Here's how the part is built. I have some questions about the finished solid (model axes, mm). A direction names the side the tool comes from. Coordinates: 2 decimals unless noted, no trailing zeros. Write each loop counter-clockwise with the first axis right and the second up, starting at its lowest first coordinate (ties: lowest second). Pieces come first, ordered by that corner, then holes.
Item 1: If I drill on line 1 (Y direction, x = -47, z = 120); line 2 (Z direction, x = -17, y = -6); line 3 (X direction, y = 11.5, z = 77.5), over which ranges is the centre line in solid material (lowest first)?
Item 2: I'm going to push flat-ended pins straight in: pin 1 Ø6 at (x, z) = (-8, -34) entering from +Y; pin 2 Ø4.5 at (x, z) = (-44.5, 119.5) entering from -Y; pin 3 Ø4.5 at (y, z) = (-14, -119.5) entering from -X; pin 4 Ø14.5 at (x, y) = (-12.5, -17) entering from -Z. Where does each tip first touch, or does it pass through?
Item 3: If we section it at B-B (x = -36.5): Please give me the cut outline in (y, z).
Item 4: If we section it at D-D (z = 7): Please give me the cut outline in (x, y), then the cut area to 3 significant figures.
Item 5: For faces 5 (the face through (-30, 32, -2)), 6 (the face through (-27, 32, -2)), 7 (the face through (2, -19, 119.25)), which set-ups out of +Z, -Z, +X, -X, +Y, -Y let a thin tool reach every point of the face, with its end or its side?
Item 6: If we section it at A-A (y = 17.5): Please give me the cut outline in (x, z).
Item 7: We'd pull the mould along Y, two halves only. Please class faces 1 (the face through (2, -19, 122.25)), 2 (the face through (14.1, -13.9, 120.8)), 3 (the face through (2, 0, -2)), 4 (the face through (-29, 60, 1)): +Y half, -Y half, draft (parallel to the pull), parting line (faces both ways), or undercut.
Item 8: If we section it at C-C (x = -12.5): Please give me the cut outline in (y, z).
from build123d import *

# Parameters (mm, degrees)
SKETCH1_W                      = 60
SKETCH1_H                      = 244.5
BASE_FLANGE1_DEPTH             = 3
EDGE_FLANGE1_STRIP_W           = 14
EDGE_FLANGE1_STRIP_H           = 3
EDGE_FLANGE1_STRIP_CUT_DEPTH   = 244.5
EDGE_FLANGE1_DEPTH             = 244.5
EDGE_FLANGE2_STRIP_W           = 14
EDGE_FLANGE2_STRIP_H           = 3
EDGE_FLANGE2_STRIP_CUT_DEPTH   = 56
EDGE_FLANGE2_STRIP_2_W         = 14
EDGE_FLANGE2_STRIP_2_H         = 3
EDGE_FLANGE2_STRIP_CUT_2_DEPTH = 56
EDGE_FLANGE2_STRIP_3_W         = 14
EDGE_FLANGE2_STRIP_3_H         = 3
EDGE_FLANGE2_STRIP_CUT_3_DEPTH = 56
EDGE_FLANGE2_STRIP_4_W         = 14
EDGE_FLANGE2_STRIP_4_H         = 3
EDGE_FLANGE2_STRIP_CUT_4_DEPTH = 56
EDGE_FLANGE2_DEPTH             = 56
EDGE_FLANGE2_BEND_DEPTH        = 56
EDGE_FLANGE2_BEND_2_DEPTH      = 56
EDGE_FLANGE2_BEND_3_DEPTH      = 56
SKETCH18_R                     = 4.6
EXTRUDE1_DEPTH                 = 261.517273899


# Sheet-metal steps are written as plain solids
with BuildPart() as part:
    # Sketch1 → Base-Flange1 (new body)
    with BuildSketch(Plane(origin=(0, 0, 0), x_dir=(1, 0, 0), z_dir=(0, 1, 0))):
        Rectangle(SKETCH1_W, SKETCH1_H)
    extrude(amount=BASE_FLANGE1_DEPTH)

    # Edge-Flange1 strip (across the edge) → Edge-Flange1 strip cut (cut)
    with BuildSketch(Plane(origin=(-30, 3, -122.25), x_dir=(1, 0, 0), z_dir=(0, 0, 1))):
        with Locations((-3, -1.5)):
            Rectangle(EDGE_FLANGE1_STRIP_W, EDGE_FLANGE1_STRIP_H)
    extrude(amount=EDGE_FLANGE1_STRIP_CUT_DEPTH, mode=Mode.SUBTRACT)

    # Edge-Flange1 section (across the edge) → Edge-Flange1 (add)
    with BuildSketch(Plane(origin=(-30, 3, -122.25), x_dir=(1, 0, 0), z_dir=(0, 0, 1))):
        with BuildLine():
            Line((0, 1), (0, 57))
            Line((0, 57), (3, 57))
            Line((3, 57), (3, 1))
            ThreePointArc((3, 1), (3.292893219, 0.292893219), (4, 0))
            Line((4, 0), (4, -3))
            ThreePointArc((4, -3), (1.171572875, -1.828427125), (0, 1))
        make_face()
    extrude(amount=EDGE_FLANGE1_DEPTH)

    # Edge-Flange2 strip (across the edge) → Edge-Flange2 strip cut (cut)
    with BuildSketch(Plane(origin=(-30, 4, 122.25), x_dir=(0, 0, -1), z_dir=(0, 1, 0))):
        with Locations((-3, -1.5)):
            Rectangle(EDGE_FLANGE2_STRIP_W, EDGE_FLANGE2_STRIP_H)
    extrude(amount=EDGE_FLANGE2_STRIP_CUT_DEPTH, mode=Mode.SUBTRACT)

    # Edge-Flange2 strip 2 (across the edge) → Edge-Flange2 strip cut 2 (cut)
    with BuildSketch(Plane(origin=(30, 0, 122.25), x_dir=(0, 0, -1), z_dir=(-1, 0, 0))):
        with Locations((-3, -1.5)):
            Rectangle(EDGE_FLANGE2_STRIP_2_W, EDGE_FLANGE2_STRIP_2_H)
    extrude(amount=EDGE_FLANGE2_STRIP_CUT_2_DEPTH, mode=Mode.SUBTRACT)

    # Edge-Flange2 strip 3 (across the edge) → Edge-Flange2 strip cut 3 (cut)
    with BuildSketch(Plane(origin=(-30, 60, -122.25), x_dir=(0, 0, 1), z_dir=(0, -1, 0))):
        with Locations((-3, -1.5)):
            Rectangle(EDGE_FLANGE2_STRIP_3_W, EDGE_FLANGE2_STRIP_3_H)
    extrude(amount=EDGE_FLANGE2_STRIP_CUT_3_DEPTH, mode=Mode.SUBTRACT)

    # Edge-Flange2 strip 4 (across the edge) → Edge-Flange2 strip cut 4 (cut)
    with BuildSketch(Plane(origin=(-26, 0, -122.25), x_dir=(0, 0, 1), z_dir=(1, 0, 0))):
        with Locations((-3, -1.5)):
            Rectangle(EDGE_FLANGE2_STRIP_4_W, EDGE_FLANGE2_STRIP_4_H)
    extrude(amount=EDGE_FLANGE2_STRIP_CUT_4_DEPTH, mode=Mode.SUBTRACT)

    # Edge-Flange2 section (across the edge) → Edge-Flange2 (add)
    with BuildSketch(Plane(origin=(-30, 4, 122.25), x_dir=(0, 0, -1), z_dir=(0, 1, 0))):
        with BuildLine():
            Line((0, 1), (0, 37))
            Line((0, 37), (3, 37))
            Line((3, 37), (3, 1))
            ThreePointArc((3, 1), (3.292893219, 0.292893219), (4, 0))
            Line((4, 0), (4, -3))
            ThreePointArc((4, -3), (1.171572875, -1.828427125), (0, 1))
        make_face()
    extrude(amount=EDGE_FLANGE2_DEPTH)

    # Edge-Flange2 section 2 (across the edge) → Edge-Flange2 bend (add)
    with BuildSketch(Plane(origin=(30, 0, 122.25), x_dir=(0, 0, -1), z_dir=(-1, 0, 0))):
        with BuildLine():
            Line((0, 1), (0, 37))
            Line((0, 37), (3, 37))
            Line((3, 37), (3, 1))
            ThreePointArc((3, 1), (3.292893219, 0.292893219), (4, 0))
            Line((4, 0), (4, -3))
            ThreePointArc((4, -3), (1.171572875, -1.828427125), (0, 1))
        make_face()
    extrude(amount=EDGE_FLANGE2_BEND_DEPTH)

    # Edge-Flange2 section 3 (across the edge) → Edge-Flange2 bend 2 (add)
    with BuildSketch(Plane(origin=(-30, 60, -122.25), x_dir=(0, 0, 1), z_dir=(0, -1, 0))):
        with BuildLine():
            Line((0, 1), (0, 37))
            Line((0, 37), (3, 37))
            Line((3, 37), (3, 1))
            ThreePointArc((3, 1), (3.292893219, 0.292893219), (4, 0))
            Line((4, 0), (4, -3))
            ThreePointArc((4, -3), (1.171572875, -1.828427125), (0, 1))
        make_face()
    extrude(amount=EDGE_FLANGE2_BEND_2_DEPTH)

    # Edge-Flange2 section 4 (across the edge) → Edge-Flange2 bend 3 (add)
    with BuildSketch(Plane(origin=(-26, 0, -122.25), x_dir=(0, 0, 1), z_dir=(1, 0, 0))):
        with BuildLine():
            Line((0, 1), (0, 37))
            Line((0, 37), (3, 37))
            Line((3, 37), (3, 1))
            ThreePointArc((3, 1), (3.292893219, 0.292893219), (4, 0))
            Line((4, 0), (4, -3))
            ThreePointArc((4, -3), (1.171572875, -1.828427125), (0, 1))
        make_face()
    extrude(amount=EDGE_FLANGE2_BEND_3_DEPTH)

    # Sketch18 → Extrude1 (cut, through all)
    with BuildSketch(Plane.XY.offset(122.25)):
        with Locations((-47, 47.5)):
            Circle(SKETCH18_R)
        with Locations((-47, 17.5)):
            Circle(SKETCH18_R)
        with Locations((-12.5, -17)):
            Circle(SKETCH18_R)
        with Locations((17.5, -17)):
            Circle(SKETCH18_R)
    extrude(amount=-EXTRUDE1_DEPTH, mode=Mode.SUBTRACT)


solid = part.part
Answer list:
1. line 1: y = 4 to 12.9, 22.1 to 42.9, 52.1 to 60
1. line 2: z = -122.25 to -119.25, 119.25 to 122.25
1. line 3: x = -30 to -27
2. pin 1: stops at y = 3
2. pin 2: stops at y = 4
2. pin 3: stops at x = -26
2. pin 4: stops at z = -122.25
3. outline: (4, -122.25) - (60, -122.25) - (60, -119.25) - (4, -119.25) - close; (4, 119.25) - (60, 119.25) - (60, 122.25) - (4, 122.25) - close
4. outline: (-30, 4) arc R4 ccw to (-26, 0) - (30, 0) - (30, 3) - (-26, 3) arc R1 cw to (-27, 4) - (-27, 60) - (-30, 60) - close
4. area: 348 mm2
5. face 5: -X, +Y, -Y
5. face 6: +Z, -Z, +X, +Y
5. face 7: +X, -X, -Y
6. outline: (-67, -122.25) - (-51.6, -122.25) - (-51.6, -119.25) - (-67, -119.25) - close; (-67, 119.25) - (-51.6, 119.25) - (-51.6, 122.25) - (-67, 122.25) - close; (-42.4, -122.25) - (-31, -122.25) arc R4 ccw to (-27, -118.25) - (-27, 118.25) arc R4 ccw to (-31, 122.25) - (-42.4, 122.25) - (-42.4, 119.25) - (-31, 119.25) arc R1 cw to (-30, 118.25) - (-30, -118.25) arc R1 cw to (-31, -119.25) - (-42.4, -119.25) - close
7. face 1: draft
7. face 2: undercut
7. face 3: -Y half
7. face 4: +Y half
8. outline: (-37, -122.25) - (-21.6, -122.25) - (-21.6, -119.25) - (-37, -119.25) - close; (-37, 119.25) - (-21.6, 119.25) - (-21.6, 122.25) - (-37, 122.25) - close; (-12.4, -122.25) - (-1, -122.25) arc R4 ccw to (3, -118.25) - (3, 118.25) arc R4 ccw to (-1, 122.25) - (-12.4, 122.25) - (-12.4, 119.25) - (-1, 119.25) arc R1 cw to (0, 118.25) - (0, -118.25) arc R1 cw to (-1, -119.25) - (-12.4, -119.25) - close
